Input: part model. Units: mm. Frame: model coordinates. Face numbers are marked on the shaded views. A direction names the side the tool comes from. Give positions to 0.01 mm unless a question says otherwise; leave off trailing zeros. Loops run counter-clockwise (first coordinate to the right, second up) from the corner with the lowest first, then second, coordinate; pieces in that order, holes last. Notation, with made-up numbers: (-18.5, 23) -> (26.5, 23) arc R25 ccw to (26.5, 62) -> close; hole circle Ø4 at (72, -11). An arc over 180 degrees is marked (long way). One line per question, with ' | ' between items.
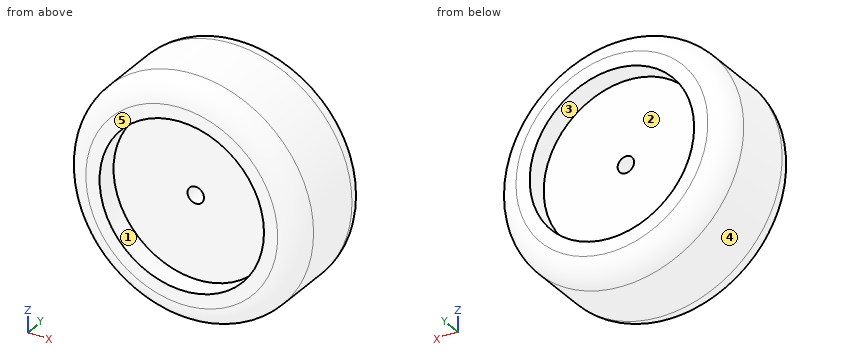
from build123d import *

# Parameters (mm, degrees)
F0_R     = 21.5
F1_DEPTH = 19
F2_R     = 4
F3_R     = 15
F4_DEPTH = 4
F5_R     = 15
F6_DEPTH = 4
F7_R     = 1.5
F8_DEPTH = 15.001


with BuildPart() as f1:
    # F0 (on Front) → F1 (new body)
    with BuildSketch(Plane.XZ):
        Circle(F0_R)
    extrude(amount=F1_DEPTH)

    # F2
    f2_edges = [f1.edges().sort_by_distance(p)[0] for p in [
        (-21.5, -19, 0),
        (-21.5, 0, 0),
    ]]
    fillet(f2_edges, radius=F2_R)

    # F3 (on face) → F4 (cut)
    with BuildSketch(Plane(origin=(0, 0, 0), x_dir=(-1, 0, 0), z_dir=(0, 1, 0))):
        Circle(F3_R)
    extrude(amount=-F4_DEPTH, mode=Mode.SUBTRACT)

    # F5 (on face) → F6 (cut)
    with BuildSketch(Plane.XZ.offset(19)):
        Circle(F5_R)
    extrude(amount=-F6_DEPTH, mode=Mode.SUBTRACT)

    # F7 (on face) → F8 (cut, through all)
    with BuildSketch(Plane.XZ.offset(15)):
        Circle(F7_R)
    extrude(amount=-F8_DEPTH, mode=Mode.SUBTRACT)


solid = f1.part
1. Pull-direction query (Z, two-part tool) for the marked faces 3, 4 and 5; classes: pulls with the +Z half, pulls with the -Z half, needs draft (parallel to the pull), parting line crosses it, or undercut.
Determined:
face 3: undercut | face 4: parting line crosses it | face 5: needs draft
2. Section query C-C (y = -6.75). Output: boundary loops of the cut face in (x, z).
Determined:
outline: circle Ø43 at (0, 0); hole circle Ø3 at (0, 0)
3. Ray query, line 1 along Z through (x, y) = (0, -8.75); line 2 along Y through (x, z) = (-9.5, -5); line 3 along Z through (x, y) = (0, -1.7). Return the intervals inside material, ascending. Write a range as from..to.
Determined:
line 1: z = -21.5..-1.5, 1.5..21.5 | line 2: y = -15..-4 | line 3: z = -20.77..-15, 15..20.77
4. Reachability of the marked faces 1 and 2 from +Z, -Z, +X, -X, +Y, -Y: full face, straight path, thin tool, end or side. Return the list, or none.
Determined:
face 1: -Y | face 2: +Y
5. Section query A-A (x = 0). Output: boundary loops of the cut face in (y, z), then the cut area to 3 significant figures.
Determined:
outline: (-19, -17.5) arc R4 ccw to (-15, -21.5) -> (-4, -21.5) arc R4 ccw to (0, -17.5) -> (0, -15) -> (-4, -15) -> (-4, -1.5) -> (-15, -1.5) -> (-15, -15) -> (-19, -15) -> close; (-19, 15) -> (-15, 15) -> (-15, 1.5) -> (-4, 1.5) -> (-4, 15) -> (0, 15) -> (0, 17.5) arc R4 ccw to (-4, 21.5) -> (-15, 21.5) arc R4 ccw to (-19, 17.5) -> close | area: 530 mm2
6. Section query B-B (z = 0). Output: boundary loops of the cut face in (x, y).
Determined:
outline: (-21.5, -15) arc R4 ccw to (-17.5, -19) -> (-15, -19) -> (-15, -15) -> (-1.5, -15) -> (-1.5, -4) -> (-15, -4) -> (-15, 0) -> (-17.5, 0) arc R4 ccw to (-21.5, -4) -> close; (1.5, -15) -> (15, -15) -> (15, -19) -> (17.5, -19) arc R4 ccw to (21.5, -15) -> (21.5, -4) arc R4 ccw to (17.5, 0) -> (15, 0) -> (15, -4) -> (1.5, -4) -> close
7. Pin query (flat end, axial travel): P1, Ø1.5, axis at x = 15, y = -2.5, coming from the +Z side; P2, Ø9, axis at x = 6, z = 2.5, coming from the +Y side; P3, Ø1, axis at y = -6, z = 13.5, coming from the -X side. Return the tip coordinate at first contact, or that it passes through.
Determined:
P1: stops at z = 15.8 | P2: stops at y = -4 | P3: stops at x = -17.12
